Design review of the part built by this model. Coordinates are the model's own, in mm. A direction names the side the tool comes from. Give positions to 0.01 mm unless a question says otherwise; leave off trailing zeros. Loops run counter-clockwise (first coordinate to the right, second up) from the corner with the lowest first, then second, coordinate; pieces in that order, holes last. Notation, with made-up numbers: (-37, 36) -> (1, 36) arc R8 cw to (1, 47) -> close; hole circle Ø11 at (-32.5, 25). An arc over 180 degrees is marked (long way). Answer in a Markdown table with one row per item. Add a question column.
(1) Consider section B-B on x = 8. Write out the cut boundary in (y, z).
(2) For faces 1 (the cylindrical face through (-18.11, 21.06, -0.03)), 2 (the cylindrical face through (4.362, 37.535, -0.225)), list the 3-axis set-ups (+Z, -Z, +X, -X, +Y, -Y) from which the entire face can be reached by the end or side of a thin tool; tool diameter is ignored.
(3) Consider section A-A on z = -0.25. Write out the cut boundary in (x, y), then the cut area to 3 significant figures.
(4) For line 1 (Y direction, x = -21, z = 0.15); line 2 (Y direction, x = -25.5, z = -0.05); line 3 (X direction, y = 15.5, z = 0.15), list the stretches that pass through material, from the lowest coordinate up.
(5) For pin 1 (5 mm diameter, centred on x = -3, y = 9, fed in from +Z); pin 2 (4 mm diameter, centred on x = -28, y = 26.5, fed in from +Z), all flat-tipped, find the tip position at first contact; note any pin that passes through.
(6) Draft analysis for pull direction Y (two halves, no side actions). For faces 3 (the cylindrical face through (-0.75, 7.6, -0.03)), 4 (the cylindrical face through (-18.5, 35.94, -0.03)), 5 (the flat face through (0, 0, 0)), state which applies: +Y half, -Y half, draft (parallel to the pull), parting line (faces both ways), or undercut.
from build123d import *

# Parameters (mm, degrees)
SKIZZE2_R = 0.75


with BuildPart() as part:
    # Austragung1: sweep along a path in Skizze1
    with BuildLine(Plane.XY) as austragung1_path:
        Line((0, 0), (0, 15))
        ThreePointArc((0, 15), (-0.840264248, 17.365573473), (-2.98450019, 18.671036644))
        Line((-2.98450019, 18.671036644), (-32.51549981, 24.828963356))
        ThreePointArc((-32.51549981, 24.828963356), (-35.499985743, 28.489659261), (-32.535734083, 32.166759053))
        Line((-32.535734083, 32.166759053), (-4.535734083, 38.166759053))
        ThreePointArc((-4.535734083, 38.166759053), (-4.145065534, 38.229131698), (-3.75, 38.25))
        Line((-3.75, 38.25), (12.25, 38.25))
    # Skizze2 → Austragung1 (sweep)
    with BuildSketch(Plane(origin=(0, 0, 0), x_dir=(1, 0, 0), z_dir=(0, 1, 0))):
        Circle(SKIZZE2_R)
    sweep(path=austragung1_path.line)


solid = part.part
Values follow:
| question | item | result |
|---|---|---|
| 1 | outline | circle Ø1.5 at (38.25, 0) |
| 2 | face 1 | none |
| 2 | face 2 | +X |
| 3 | outline | (-32.68, 32.86) arc R4.46 ccw to (-32.66, 24.14) -> (-3.13, 17.98) arc R3.04 cw to (-0.71, 15) -> (-0.71, 0) -> (0.71, 0) -> (0.71, 15) arc R4.46 ccw to (-2.84, 19.36) -> (-32.37, 25.52) arc R3.04 cw to (-32.39, 31.48) -> (-4.39, 37.48) arc R3.04 cw to (-3.75, 37.54) -> (12.25, 37.54) -> (12.25, 38.96) -> (-3.75, 38.96) arc R4.46 ccw to (-4.68, 38.86) -> close |
| 3 | area | 150 mm2 |
| 4 | line 1 | 21.68 to 23.18, 33.89 to 35.39 |
| 4 | line 2 | 22.6 to 24.13, 32.91 to 34.44 |
| 4 | line 3 | -0.78 to 0.71 |
| 5 | pin 1 | z = 0.56 |
| 5 | pin 2 | z = 0.5 |
| 6 | face 3 | draft |
| 6 | face 4 | undercut |
| 6 | face 5 | -Y half |
